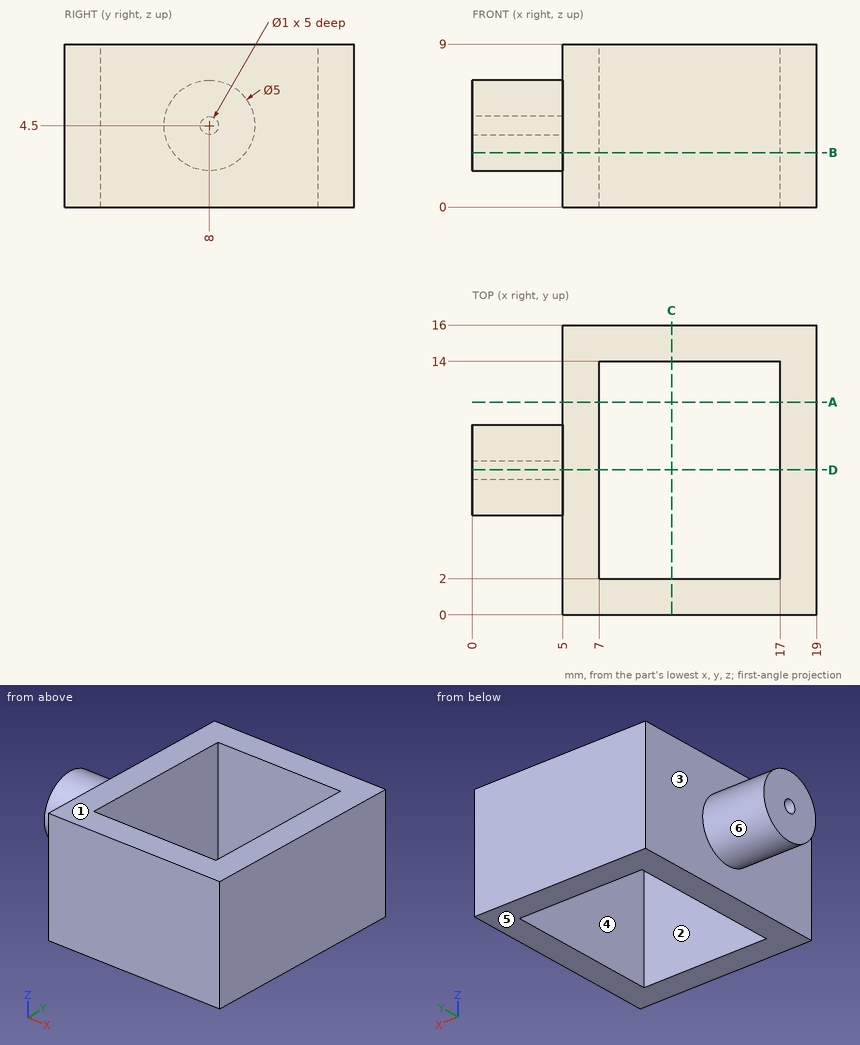
Answer from the drawing. Dimensions are ordinates in mm from the lowest x, y and z of the part. A direction names the side the tool comes from. Coordinates: 2 decimals unless noted, no trailing zeros. Loops run counter-clockwise (first coordinate to the right, second up) from the corner with the lowest first, then second, coordinate; pieces in that order, holes last. Notation, with made-up numbers: (72.25, -6) - (113.25, -6) arc R7 ccw to (113.25, -1) - close; hole circle Ø2 at (60, -30.75). An arc over 180 degrees is marked (long way). Use a Markdown table: item, result.
Item 1: For the marked faces 4, 5 and 6, determine the directions among +Z, -Z, +X, -X, +Y, -Y from which every point of the face is accessible in a straight line to the end or side of a thin tool.
Evaluation:
| item | result |
|---|---|
| face 4 | +Z, -Z |
| face 5 | -Z, +X, -X, +Y, -Y |
| face 6 | -X |
Item 2: Consider probe 1 along Y at (x, z) = (1.2, 4.5); probe 2 along X at (y, z) = (8.75, 7); probe 3 along Y at (x, z) = (11.5, 1.75). Determine where each line is inside the solid, lowest interval first. Write a range as from..to.
Evaluation:
| item | result |
|---|---|
| probe 1 | y = 5.5..7.5, 8.5..10.5 |
| probe 2 | x = 5..7, 17..19 |
| probe 3 | y = 0..2, 14..16 |
Item 3: The mould has two halves that part along X. Classify the marked faces 1, 2 and 3: +X half, -X half, draft (parallel to the pull), parting line (faces both ways), or undercut.
Evaluation:
| item | result |
|---|---|
| face 1 | draft |
| face 2 | undercut |
| face 3 | -X half |
Item 4: Find section A-A, the plane y = 11.75. Determine the outline of the cut face in (x, z), and give its area (3 significant figures).
Evaluation:
| item | result |
|---|---|
| outline | (5, 0) - (7, 0) - (7, 9) - (5, 9) - close; (17, 0) - (19, 0) - (19, 9) - (17, 9) - close |
| area | 36.0 mm2 |
Item 5: Find section D-D, the plane y = 8. Determine the outline of the cut face in (x, z).
Evaluation:
| item | result |
|---|---|
| outline | (0, 2) - (5, 2) - (5, 0) - (7, 0) - (7, 9) - (5, 9) - (5, 7) - (0, 7) - (0, 5) - (5, 5) - (5, 4) - (0, 4) - close; (17, 0) - (19, 0) - (19, 9) - (17, 9) - close |
Item 6: Find section C-C, the plane x = 11. Determine the outline of the cut face in (y, z), and give its area (3 significant figures).
Evaluation:
| item | result |
|---|---|
| outline | (0, 0) - (2, 0) - (2, 9) - (0, 9) - close; (14, 0) - (16, 0) - (16, 9) - (14, 9) - close |
| area | 36.0 mm2 |
Item 7: Find section B-B, the plane z = 3. Determine the outline of the cut face in (x, y), and give its area (3 significant figures).
Evaluation:
| item | result |
|---|---|
| outline | (0, 6) - (5, 6) - (5, 0) - (19, 0) - (19, 16) - (5, 16) - (5, 10) - (0, 10) - close; hole (7, 2) - (17, 2) - (17, 14) - (7, 14) - close |
| area | 124 mm2 |
Item 8: Given pin 1 Ø5 at (x, z) = (12, 6.5) entering from -Y; pin 2 Ø0.8 at (y, z) = (8, 4.5) entering from -X, each flat-ended and moving along its own axis, determine where each tip first touches the part or whether it passes through.
Evaluation:
| item | result |
|---|---|
| pin 1 | stops at y = 0 |
| pin 2 | stops at x = 5 |
